Autodesk Inventor part; units mm, degrees
ref_plane "MSC_PF1" through (0, 0, 0) normal (1, 0, 0) x (0, 1, 0)
ref_plane "MSC_PT1" through (2.675, 0, -0.685) normal (0, 0, -1) x (-1, 0, 0)
ref_plane "YZ Plane" through (0, 0, 0) normal (1, 0, 0) x (0, 1, 0)
sketch "Esquisse2" plane through (0, 0, 0) normal (0, 1, 0) x (-1, 0, 0)
  line L0 (0, -6) -> (-1.5, -6)
  line L1 (0, 0) -> (0, -6)
  line L2 (-2.675, 0) -> (0, 0)
  line L3 (-2.675, -0.685) -> (-2.675, 0)
  line L4 (-1.5, -1.86) -> (-2.675, -0.685)
  line L5 (-1.5, -6) -> (-1.5, -1.86)
  line L6 (0, 0) -> (0, -6)
  dimension "d2" = 45
  dimension "d4" = 1.5
  dimension "d6" = 2.675
  dimension "d8" = 1.86
  dimension "d10" = 6
revolve "Révolution1" add sketch "Esquisse2" angle 360 about axis through (0, 0, 0) along (0, 0, -1)
fillet "Congé1" radius 0.25 1 edges at (-1.5, 0, -1.86)
chamfer "Chanfrein1" distance 0.25 angle 45 1 edges at (-1.5, 0, -6)
sketch "Esquisse4" plane through (0, 0, 0) normal (0, 0, 1) x (1, 0, 0)
  circle A0 centre (0, 0) radius 2.675
  circle A1 centre (0, 0) radius 1 construction
  line L0 (-1, -0.5774) -> (-1, 0.5774)
  line L1 (-1, 0.5774) -> (0, 1.1547)
  line L2 (0, 1.1547) -> (1, 0.5774)
  line L3 (1, 0.5774) -> (1, -0.5774)
  line L4 (1, -0.5774) -> (0, -1.1547)
  line L5 (0, -1.1547) -> (-1, -0.5774)
  dimension "d27" = 2
extrude "Extrusion1" cut sketch "Esquisse4" against normal blind 1.1 contours L0 L1 L2 L3 L4 L5
sketch "Esquisse5" plane through (0, 0, 0) normal (0, 0, 1) x (1, 0, 0)
  circle A0 centre (0, 0) radius 2.675
  circle A1 centre (0, 0) radius 1.01
  dimension "d38" = 2.02
extrude "Extrusion2" cut sketch "Esquisse5" against normal blind 1.1 contours A1
thread "Filetage1"
ref_plane "MSC_PF1" through (0, 0, 0) normal (1, 0, 0) x (0, 1, 0)
ref_plane "MSC_PT1" through (2.675, 0, -0.685) normal (0, 0, -1) x (-1, 0, 0)
equation "\"d4\" = 0.5 * NND"
equation "\"d6\" = 0.5 * ParA"
equation "\"d8\" = ParH"
equation "\"d10\" = NLG"
equation "\"d27\" = ParJ"
equation "\"d39\" = Tt"
equation "\"d24\" = Rr"
equation "\"d25\" = 0.5 * PTC"
equation "\"d26\" = 0.5 * PTC"
equation "\"d28\" = Tt"
equation "\"d31\" = Lt"
equation "\"d38\" = 1.01 * ParJ"
equation "\"NND\" = 3"
equation "\"NLG\" = 6"
equation "\"PTC\" = 0.5"
equation "\"ParA\" = 5.35"
equation "\"ParH\" = 1.86"
equation "\"ParJ\" = 2"
equation "\"Tt\" = 1.1"
equation "\"Rr\" = 0.25"
equation "\"msp_e\" = 0.288675 * ParJ"
equation "\"Lt\" = 3.14"
equation "\"THREADDIA\" = NND"
properties part number "ASME/ANSI B18.3.5M - M3x6(2)" material "Acier, doux"
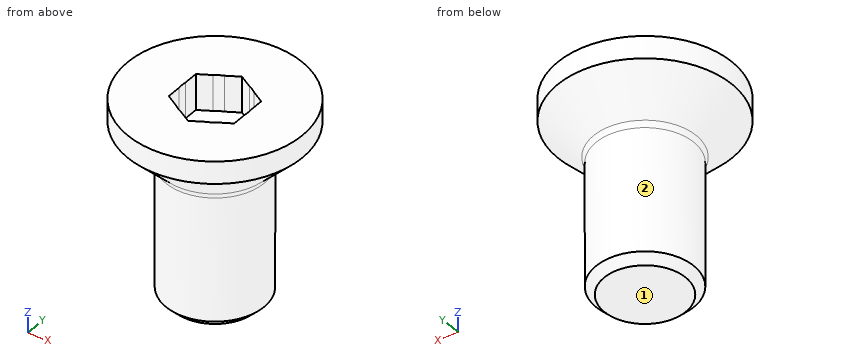
Check sheet for the modelled part. Datum: model origin and axes. Units: mm. Face numbers are marked on the shaded views. A direction names the side the tool comes from. Round coordinates to 2 decimals unless told otherwise and drop trailing zeros. Order: outer loops, then holes, each group sorted by start corner. A loop starts at its lowest first (then second) coordinate and runs counter-clockwise, first axis right, second up.
(1) Cross-section at B-B, the plane z = -1.45. Enter the section's corners in (x, y), and give its area (3 significant figures).
(2) Access from +Z, -Z, +X, -X, +Y, -Y to the whole of each face (thin tool, end or side, straight path). Record for the marked faces 1 and 2.
(3) Cross-section at A-A, the plane z = -4.9. Enter the section's corners in (x, y), and give its area (3 significant figures).
(4) Scan lines: probe 1 along Z at (x, y) = (-0.2, -1); probe 2 along X at (y, z) = (-0.05, -3.15); probe 3 along Y at (x, z) = (0.8, -0.3). Record each from-to range of solid material in increasing order.
(5) Go/stop test with flat-tipped pins: P1, Ø1, axis at y = -1.5, z = -2, coming from the -X side; P2, Ø1, axis at x = 0, z = -1.5, coming from the +Y side; P3, Ø1.5, axis at y = 1.5, z = -5, coming from the +X side. Record where each tip stops, or that it passes through.
Check sheet entries:
1. outline: circle Ø3.82 at (0, 0)
1. area: 11.5 mm2
2. face 1: -Z, +X, -X, +Y, -Y
2. face 2: -Z
3. outline: circle Ø3 at (0, 0)
3. area: 7.07 mm2
4. probe 1: z = -6 to -1.1
4. probe 2: x = -1.5 to 1.5
4. probe 3: y = -2.55 to -0.69, 0.69 to 2.55
5. P1: stops at x = -1.29
5. P2: stops at y = 2.36
5. P3: stops at x = 1.3
